```python
from build123d import *

# Parameters (mm, degrees)
FILLET2_R = 1.27


with BuildPart() as part:
    # Sketch1 → Revolve1 (revolve)
    with BuildSketch(Plane.YZ, mode=Mode.PRIVATE) as revolve1_sk:
        Polygon((10.16, 0), (10.16, 17.78), (53.34, 17.78), (38.1, 12.7), (38.1, 5.08), (53.357021735, 0), align=None)
    revolve(revolve1_sk.sketch.rotate(Axis((0, 0, 0), (0, 0, 1)), 90), axis=Axis((0, 0, 0), (0, 0, 1)))

    # Fillet2
    fillet2_edges = [part.edges().sort_by_distance(p)[0] for p in [
        (53.34, 0, 17.78),
        (53.357021735, 0, 0),
    ]]
    fillet(fillet2_edges, radius=FILLET2_R)


solid = part.part
```
Geometry: final body of the model. Coordinates: model frame, mm. A direction names the side the tool comes from. Coordinates: 2 decimals unless noted, no trailing zeros. Order: outer loops, then holes, each group sorted by start corner. A loop starts at its lowest first (then second) coordinate and runs counter-clockwise, first axis right, second up. Notation, with made-up numbers: (7.25, -36) - (47.25, -36) arc R21 cw to (47.25, -32) - close; hole circle Ø9 at (58.25, 77). An arc over 180 degrees is marked (long way). Return JSON: item names as keys, results as strings. Group by question number.
1. Cut plane A-A (x = 0). Output: boundary loops of the cut face in (y, z).
2. Cut plane C-C (z = 8.25). Output: boundary loops of the cut face in (x, y), plus the area to 3 significant figures.
3. Pull-direction query (Z, two-part tool) for faces 1 (the face through (-17.807, 34.235, 4.917)), 2 (the face through (-1, -11, 17.78)), 3 (the face through (1.323, -10.074, 9.014)); classes: pulls with the +Z half, pulls with the -Z half, needs draft (parallel to the pull), parting line crosses it, or undercut.
4. Pin query (flat end, axial travel): pin 1 (2 mm diameter, centred on y = -22, z = 10, fed in from +X); pin 2 (10 mm diameter, centred on y = 36, z = 12.5, fed in from +X); pin 3 (3 mm diameter, centred on x = -28.5, z = 8.5, fed in from +Y). Return the tip coordinate at first contact, or that it passes through.
5. Material intervals for line 1 along Z through (x, y) = (18, 35.5); line 2 along Z through (x, y) = (32, -24); line 3 along Y through (x, z) = (-4, 15.5), sorted ascending. Write a range as [from, to].
6. Set-up query: faces 4 (the face through (1, -11, 0)), 5 (the face through (8.259, 37.194, 8.837)). Return all of +Z, -Z, +X, -X, +Y, -Y with unobstructed straight access to the full face (end or side cutting, diameter ignored); none if empty.
Resolved:
{
 "1": {"outline": "(-45.92, 2.47) arc R1.27 ccw to (-45.52, 0) - (-10.16, 0) - (-10.16, 17.78) - (-45.51, 17.78) arc R1.27 ccw to (-45.92, 15.31) - (-38.1, 12.7) - (-38.1, 5.08) - close; (10.16, 0) - (45.52, 0) arc R1.27 ccw to (45.92, 2.47) - (38.1, 5.08) - (38.1, 12.7) - (45.92, 15.31) arc R1.27 ccw to (45.51, 17.78) - (10.16, 17.78) - close"},
 "2": {"outline": "circle Ø76.2 at (0, 0); hole circle Ø20.32 at (0, 0)", "area": "4,240 mm²"},
 "3": {"face 1": "undercut", "face 2": "pulls with the +Z half", "face 3": "needs draft"},
 "4": {"pin 1": "stops at x = 31.79", "pin 2": "stops at x = 33.6", "pin 3": "stops at y = 26.88"},
 "5": {"line 1": "z = [0, 4.51], [13.27, 17.78]", "line 2": "z = [0, 4.45], [13.33, 17.78]", "line 3": "y = [-46.11, -9.34], [9.34, 46.11]"},
 "6": {"face 4": "-Z, +X, -X, +Y, -Y", "face 5": "none"}
}
